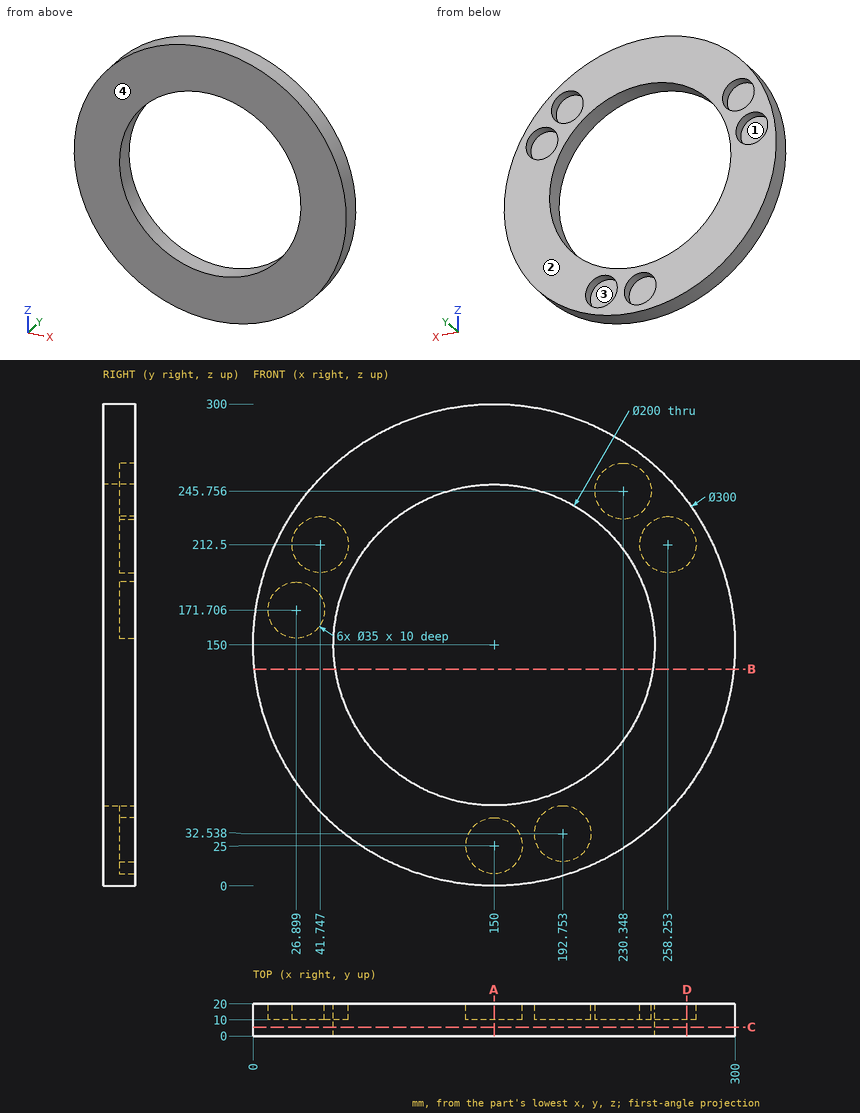
Part print with two shaded views. Sizes in mm from the minimum x, y, z corner. A direction names the side the tool comes from. Round coordinates to 2 decimals unless told otherwise and drop trailing zeros. Loops run counter-clockwise (first coordinate to the right, second up) from the corner with the lowest first, then second, coordinate; pieces in that order, holes last. Notation, with made-up numbers: (59.5, 73) - (65.5, 73) arc R37 cw to (65.5, 109) - close; hole circle Ø8 at (60.5, 34). An arc over 180 degrees is marked (long way). Answer as a JSON object with one key per item and string values.
Item 1: Band-saw the part on C-C on y = 5.5. List the corners of the cut face in (x, z).
Output:
{"outline": "circle Ø300 at (150, 150); hole circle Ø200 at (150, 150)"}
Item 2: Wall check: L1, parallel to X at y = 9.25, z = 150; L2, parallel to Z at x = 148.5, y = 13 (1 decimal); L3, parallel to X at y = 14.5, z = 212.5 (1 decimal). Give the ranges that are in metal, low to high.
Output:
{"L1": "0 to 50, 250 to 300", "L2": "0 to 7.6, 42.4 to 50, 250 to 300", "L3": "13.6 to 24.2, 59.2 to 71.9, 228.1 to 240.8, 275.8 to 286.4"}
Item 3: Tool access for the marked faces 3 and 4: list every direction of +Z, -Z, +X, -X, +Y, -Y with a clear straight run to the whole face (end or side of a thin tool).
Output:
{"face 3": "+Y", "face 4": "+Z, -Z, +X, -X, -Y"}
Item 4: Band-saw the part on D-D on x = 270. List the corners of the cut face in (y, z), plus the area to 3 significant figures.
Output:
{"outline": "(0, 60) - (20, 60) - (20, 199.53) - (10, 199.53) - (10, 225.47) - (20, 225.47) - (20, 240) - (0, 240) - close", "area": "3,340 mm2"}
Item 5: Band-saw the part on B-B on z = 135. List the corners of the cut face in (x, y), plus the area to 4 significant figures.
Output:
{"outline": "(0.75, 0) - (51.13, 0) - (51.13, 20) - (0.75, 20) - close; (248.87, 0) - (299.25, 0) - (299.25, 20) - (248.87, 20) - close", "area": "2,015 mm2"}
Item 6: Pin check, flat tips, straight feed: pin 1 (10.5 mm diameter, centred on x = 227.5, z = 246.5, fed in from +Y); pin 2 (2 mm diameter, centred on y = 10.5, z = 102.5, fed in from +X); pin 3 (5 mm diameter, centred on y = 8.5, z = 196, fed in from -X). Stop position of each tip, or through.
Output:
{"pin 1": "y = 10", "pin 2": "x = 292.61", "pin 3": "x = 6.45"}
Item 7: Pull direction X, two halves, no side cores. Call the marked faces 1 and 2: pulls with the +X half, pulls with the -X half, needs draft (parallel to the pull), parting line crosses it, or undercut.
Output:
{"face 1": "undercut", "face 2": "needs draft"}
Item 8: Band-saw the part on A-A on x = 150. List the corners of the cut face in (y, z), plus the area to 3 significant figures.
Output:
{"outline": "(0, 0) - (20, 0) - (20, 7.5) - (10, 7.5) - (10, 42.5) - (20, 42.5) - (20, 50) - (0, 50) - close; (0, 250) - (20, 250) - (20, 300) - (0, 300) - close", "area": "1,650 mm2"}
